from build123d import *

# Parameters (mm, degrees)
F0_W           = 190
F0_H           = 1000
F1_DEPTH       = 15
F2_D           = 75
F2_DEPTH       = 15
F2_CBORE_D     = 104
F2_CBORE_DEPTH = 4
F3_D           = 145
F3_DEPTH       = 15
F3_CBORE_D     = 171
F3_CBORE_DEPTH = 6.5
F4_D           = 145
F4_DEPTH       = 15
F4_CBORE_D     = 171
F4_CBORE_DEPTH = 6.5
F5_D           = 4
F5_DEPTH       = 15
F6_SIZE        = 1.5


with BuildPart() as f1:
    # F0 (on Front) → F1 (new body)
    with BuildSketch(Plane.XZ):
        Rectangle(F0_W, F0_H)
    extrude(amount=-F1_DEPTH)

    # F2
    with Locations(Plane.XZ):
        with Locations((0, 360)):
            CounterBoreHole(F2_D / 2, F2_CBORE_D / 2, F2_CBORE_DEPTH, depth=F2_DEPTH)

    # F3
    with Locations(Plane.XZ):
        with Locations((0, 200)):
            CounterBoreHole(F3_D / 2, F3_CBORE_D / 2, F3_CBORE_DEPTH, depth=F3_DEPTH)

    # F4
    with Locations(Plane.XZ):
        with Locations((0, 5)):
            CounterBoreHole(F4_D / 2, F4_CBORE_D / 2, F4_CBORE_DEPTH, depth=F4_DEPTH)

    # F5
    with Locations(Plane.XZ):
        with Locations((-56.214989, 256.214989), (56.214989, 256.214989), (56.214989, 143.785011), (-56.214989, 143.785011), (-56.947881, 63.257827), (55.482097, 63.257827), (55.482097, -49.172151), (-56.947881, -49.172151), (-32.880465, 392.880465), (32.880465, 392.880465), (32.880465, 327.119535), (-32.880465, 327.119535)):
            Hole(F5_D / 2, depth=F5_DEPTH)

    # F6
    f6_edges = [f1.edges().sort_by_distance(p)[0] for p in [
        (-95, 0, 0),
        (0, 0, 500),
        (95, 0, 0),
        (0, 0, -500),
        (-95, 7.5, -500),
        (-95, 15, 0),
        (0, 15, -500),
        (95, 7.5, -500),
        (95, 15, 0),
        (-95, 7.5, 500),
        (0, 15, 500),
        (95, 7.5, 500),
    ]]
    chamfer(f6_edges, length=F6_SIZE)


solid = f1.part
Geometry: final body of the model. Coordinates: model frame, mm. A direction names the side the tool comes from. Coordinates: 2 decimals unless noted, no trailing zeros. Order: outer loops, then holes, each group sorted by start corner. A loop starts at its lowest first (then second) coordinate and runs counter-clockwise, first axis right, second up. Notation, with made-up numbers: (56.25, 37) - (90.25, 37) arc R23 ccw to (90.25, 53) - close; hole circle Ø1 at (23, -5). An arc over 180 degrees is marked (long way). Use one line per item in the form item = value.
1) Mould query, pull axis Z, two halves, no side actions, for faces 1 (the face through (34.4, 4, 375.7)), 2 (the face through (-1, 0, -104)). Classes: +Z half, -Z half, draft (parallel to the pull), parting line (faces both ways), or undercut.
Solutions:
face_1 = undercut
face_2 = draft
2) Section C-C (z = 200). Return loops of the section in (x, y), then the cut area to 4 significant figures.
Solutions:
outline = (-95, 1.5) - (-93.5, 0) - (-85.5, 0) - (-85.5, 6.5) - (-72.5, 6.5) - (-72.5, 15) - (-93.5, 15) - (-95, 13.5) - close; (72.5, 6.5) - (85.5, 6.5) - (85.5, 0) - (93.5, 0) - (95, 1.5) - (95, 13.5) - (93.5, 15) - (72.5, 15) - close
area = 501.5 mm^2
3) Section B-B (x = 0). State how many separate pieces and enclosed holes the cut face has, then the cut area to 3 significant figures.
Solutions:
separate_pieces = 4
enclosed_holes = 0
area = 9,070 mm^2
4) Set-up query: faces 3 (the face through (-11.273, 1.972, 309.237)), 4 (the face through (-17.3, 9.58, 326.73)). Return all of +Z, -Z, +X, -X, +Y, -Y with unobstructed straight access to the full face (end or side cutting, diameter ignored); none if empty.
Solutions:
face_3 = -Y
face_4 = +Y, -Y
5) Ray query, L1, parallel to Z at x = 0, y = 10.75; L2, parallel to Z at x = 49, y = 6.25; L3, parallel to Z at x = -51, y = 12.75. Return the intervals inside material, ascending.
Solutions:
L1 = -500 to -67.5, 77.5 to 127.5, 272.5 to 322.5, 397.5 to 500
L2 = -500 to -65.07, 75.07 to 129.93, 270.07 to 500
L3 = -500 to -46.53, 56.53 to 148.47, 251.53 to 500
6) Section A-A (z = 360). Return loops of the section in (x, y).
Solutions:
outline = (-95, 1.5) - (-93.5, 0) - (-52, 0) - (-52, 4) - (-37.5, 4) - (-37.5, 15) - (-93.5, 15) - (-95, 13.5) - close; (37.5, 4) - (52, 4) - (52, 0) - (93.5, 0) - (95, 1.5) - (95, 13.5) - (93.5, 15) - (37.5, 15) - close
7) Pin query (flat end, axial travel): pin 1 (3.5 mm diameter, centred on x = -56.21, z = 143.79, fed in from +Y). Return the tip coordinate at first contact, or that it passes through.
Solutions:
pin_1 = through
